Source: three-view drawing plus pictorial views. Frame: mm from the lowest corner of the part. A direction names the side the tool comes from. Give positions to 0.01 mm unless a question says otherwise; leave off trailing zeros. Order: outer loops, then holes, each group sorted by start corner. A loop starts at its lowest first (then second) coordinate and runs counter-clockwise, first axis right, second up. Notation, with made-up numbers: M -4,33 L 46,33 A23 cw 46,59 Z; hole C 26.25,-14 d10. An arc over 180 degrees is marked long. One line per question, with ' | ' between items. Start each with the question number.
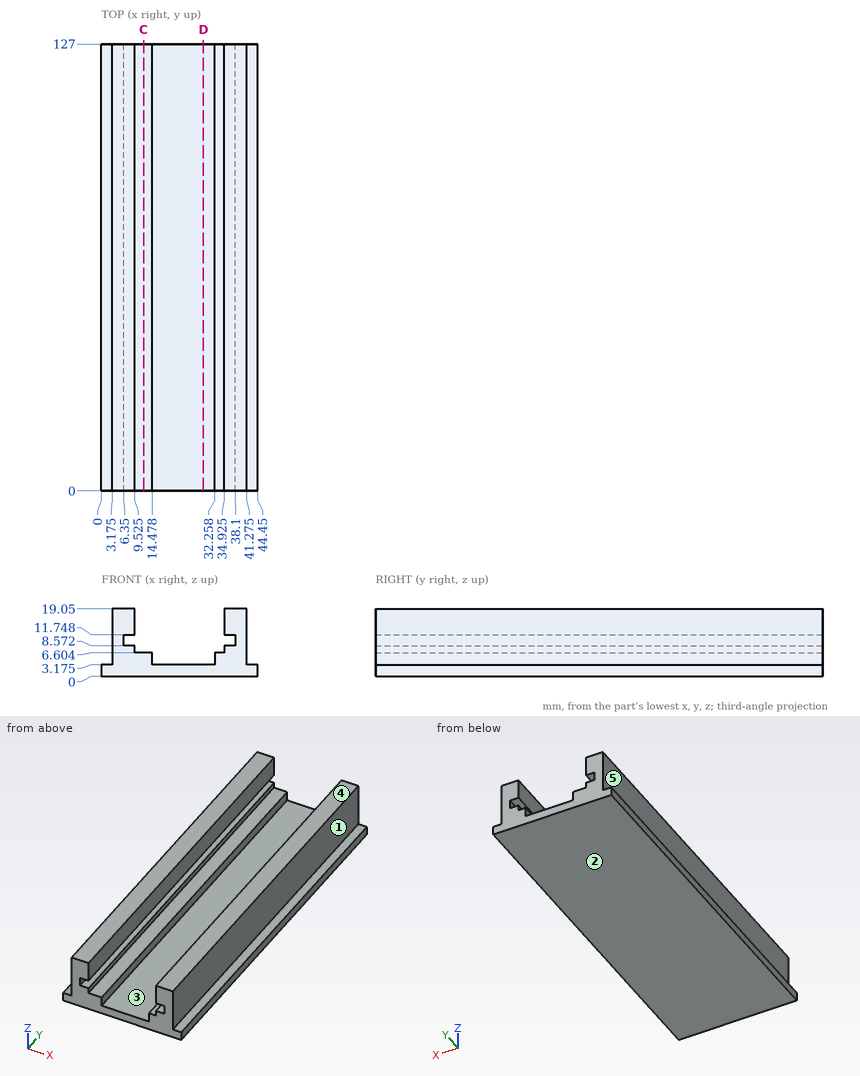
Item 1: Mould query, pull axis X, two halves, no side actions, for the marked faces 1, 2 and 3. Classes: pulls with the +X half, pulls with the -X half, needs draft (parallel to the pull), parting line crosses it, or undercut.
Item 2: Line query: line 1 (X direction, y = 113, z = 14.5) (1 decimal); line 2 (X direction, y = 108, z = 3.25) (1 decimal); line 3 (Z direction, x = 7.5, y = 92). Output: solid intervals per line, ascending.
Item 3: Cut plane C-C on x = 12. Return the cut outline in (y, z) (1 decimal).
Item 4: Cut plane D-D on x = 29. Return the cut outline in (y, z) (1 decimal).
Item 5: Pin query (flat end, axial travel): pin 1 Ø1.5 at (x, z) = (16, 7) entering from +Y; pin 2 Ø5.5 at (x, y) = (26.5, 33) entering from +Z (1 decimal); pin 3 Ø0.6 at (y, z) = (71.5, 7.5) entering from +X (1 decimal); pin 4 Ø2 at (y, z) = (64.5, 7) entering from -X (1 decimal). Return the tip coordinate at first contact, or that it passes through.
Item 6: Reachability of the marked faces 4 and 5 from +Z, -Z, +X, -X, +Y, -Y: full face, straight path, thin tool, end or side. Return the list, or none.
Results are:
1) face 1: pulls with the +X half | face 2: needs draft | face 3: undercut
2) line 1: x = 3.2 to 9.5, 34.9 to 41.3 | line 2: x = 3.2 to 14.5, 32.3 to 41.3 | line 3: z = 0 to 8.57, 11.75 to 19.05
3) outline: M 0,0 L 127,0 L 127,6.6 L 0,6.6 Z
4) outline: M 0,0 L 127,0 L 127,3.2 L 0,3.2 Z
5) pin 1: passes through | pin 2: stops at z = 3.2 | pin 3: stops at x = 41.3 | pin 4: stops at x = 3.2
6) face 4: +Z, +X, -X, +Y, -Y | face 5: +Z, -X, +Y, -Y
